```python
from build123d import *

# Parameters (mm, degrees)
SKETCH2_R           = 14.2875
SKETCH2_R_2         = 4.064
SKETCH2_R_3         = 6.35
BOSS_EXTRUDE1_DEPTH = 6.35


with BuildPart() as part:
    # Sketch2 → Boss-Extrude1 (new body)
    with BuildSketch(Plane(origin=(0, 0, 0), x_dir=(1, 0, 0), z_dir=(0, 1, 0))):
        with BuildLine():
            Line((31.75, -78.393028047), (31.75, 117.475))
            ThreePointArc((31.75, 117.475), (27.49630657, 133.35), (15.875, 144.97130657))
            add(Edge.make_bspline(
                [(-11.426385325, 153.835795689), (1.224450482, 152.855976047), (15.875, 144.97130657)],
                knots=[0, 0, 0, 1, 1, 1], degree=2))
            add(Edge.make_bspline(
                [(-64.783506655, 184.207168681), (-52.423507121, 162.771572898), (-33.18367174, 151.627706727), (-11.426385325, 153.835795689)],
                knots=[0, 0, 0, 0, 1, 1, 1, 1], degree=3))
            add(Edge.make_bspline(
                [(-85.86133431, 203.70880657), (-72.386286962, 196.104383794), (-64.783506655, 184.207168681)],
                knots=[0, 0, 0, 1, 1, 1], degree=2))
            ThreePointArc((-85.86133431, 203.70880657), (-129.23264088, 192.0875), (-117.61133431, 148.71619343))
            Line((-117.61133431, 148.71619343), (-57.15, 113.808825791))
            ThreePointArc((-57.15, 113.808825791), (-38.555909488, 95.214735278), (-31.75, 69.814735278))
            Line((-31.75, 69.814735278), (-31.75, -18.272918452))
            Line((-31.75, -18.272918452), (-31.75, -139.7))
            ThreePointArc((-31.75, -139.7), (0, -171.45), (31.75, -139.7))
            Line((31.75, -139.7), (31.75, -78.393028047))
        make_face()
        with Locations(Location((0, 0, 0), (0, 0, 270))):
            Circle(SKETCH2_R, mode=Mode.SUBTRACT)
        with Locations(Location((0, -88.9, 0), (0, 0, 270))):
            Circle(SKETCH2_R, mode=Mode.SUBTRACT)
        with Locations(Location((0, 117.475, 0), (0, 0, 270))):
            Circle(SKETCH2_R, mode=Mode.SUBTRACT)
        with Locations(Location((-101.73633431, 176.2125, 0), (0, 0, 270))):
            Circle(SKETCH2_R, mode=Mode.SUBTRACT)
        with Locations(Location((-50.868167155, 146.84375, 0), (0, 0, 270))):
            Circle(SKETCH2_R_2, mode=Mode.SUBTRACT)
        with Locations(Location((0, 58.7375, 0), (0, 0, 270))):
            Circle(SKETCH2_R_2, mode=Mode.SUBTRACT)
        with Locations(Location((0, -152.4, 0), (0, 0, 270))):
            Circle(SKETCH2_R_3, mode=Mode.SUBTRACT)
    extrude(amount=BOSS_EXTRUDE1_DEPTH)


solid = part.part
```
Here's how the part is built. I have some questions about the finished solid (model axes, mm). A direction names the side the tool comes from. Give positions to 0.01 mm unless a question says otherwise; leave off trailing zeros. Write each loop counter-clockwise with the first axis right and the second up, starting at its lowest first coordinate (ties: lowest second). Pieces come first, ordered by that corner, then holes. Notation, with made-up numbers: M 46.5,13.5 L 67.5,13.5 A14 ccw 67.5,24.5 Z; hole C 77,46 d1. An arc over 180 degrees is marked long. Put each result on its own line as item: value. Start each with the question number.
Item 1: If we section it at D-D, the plane y = 4.75: Count the separate pieces of the cut face and the enclosed holes in it, then the cut area to 3 significant figures.
Item 2: If we section it at C-C, the plane z = 60: Write out the boundary of the cut face in (x, y), then the cut area to 3 significant figures.
Item 3: On a 3-axis mill with a long thin cutter (end or side, diameter ignored), from which of +Z, -Z, +X, -X, +Y, -Y can I reach the whole of each face in a straight line? I mean faces 4 (the flat face through (-31.75, 3, 33)), 5 (the cylindrical face through (1.907, 3.131, 158.457)). Say none if no direction works.
Item 4: Thinking about a two-plate mould opening in Z: for faces 1 (the cylindrical face through (0.179, 3.131, -62.798)), 2 (the cylindrical face through (-128.877, 3.131, -192.688)), 3 (the cylindrical face through (27.61, 3.13, -133.15)), which applies, +Z half, -Z half, draft (parallel to the pull), parting line (faces both ways), or undercut?
Item 5: If we section it at A-A, the plane z = 0: Write out the boundary of the cut face in (x, y), then the cut area to 3 significant figures.
Item 6: If we section it at B-B, the plane x = -98: Write out the boundary of the cut face in (y, z).
Item 7: Will these pins go through, and if not, where does the flat tip stop? pin 1 (3 mm diameter, centred on x = -94.5, y = 2.5, fed in from +Z); pin 2 (1.5 mm diameter, centred on x = -33.5, y = 5.5, fed in from -Z); pin 3 (1.9 mm diameter, centred on y = 4.5, z = 73.5, fed in from -X).
Item 8: I need wall thicknesses on L1, parallel to X at y = 5, z = 88.9; L2, parallel to X at y = 4.5, z = -175; L3, parallel to Z at x = -108.5, y = 4. Which ranges of each line are inside material? Lowest first, please. Write a range as from..to.
Values:
1. separate pieces: 1
1. enclosed holes: 7
1. area: 23,400 mm²
2. outline: M -31.75,0 L 31.75,0 L 31.75,6.35 L -31.75,6.35 Z
2. area: 403 mm²
3. face 4: +Z, -X, +Y, -Y
3. face 5: +Y, -Y
4. face 1: undercut
4. face 2: parting line
4. face 3: -Z half
5. outline: M -31.75,0 L -14.29,0 L -14.29,6.35 L -31.75,6.35 Z; M 14.29,0 L 31.75,0 L 31.75,6.35 L 14.29,6.35 Z
5. area: 222 mm²
6. outline: M 0,-207.74 L 6.35,-207.74 L 6.35,-190 L 0,-190 Z; M 0,-162.42 L 6.35,-162.42 L 6.35,-137.39 L 0,-137.39 Z
7. pin 1: z = -134.51
7. pin 2: z = -156.69
7. pin 3: x = -31.75
8. L1: -31.75..-14.29, 14.29..31.75
8. L2: -133.46..-115.97, -87.5..-58.56
8. L3: -207.23..-188.8, -163.63..-143.46
